from build123d import *

# Parameters (mm, degrees)
F0_R     = 6.5
F1_DEPTH = 50
F2_R     = 5.75
F3_DEPTH = 15
F4_R     = 4
F5_DEPTH = 4.5
F6_R     = 1


with BuildPart() as f1:
    # F0 (on Front) → F1 (new body)
    with BuildSketch(Plane.XZ):
        Circle(F0_R)
    extrude(amount=F1_DEPTH)

    # F2 (on face) → F3 (join)
    with BuildSketch(Plane.XZ.offset(50)):
        Circle(F2_R)
    extrude(amount=F3_DEPTH)

    # F4 (on face) → F5 (join)
    with BuildSketch(Plane.XZ.offset(65)):
        Circle(F4_R)
    extrude(amount=F5_DEPTH)

    # F6
    f6_edges = [f1.edges().sort_by_distance(p)[0] for p in [
        (-4, -69.5, 0),
        (-5.75, -65, 0),
        (-6.5, 0, 0),
    ]]
    fillet(f6_edges, radius=F6_R)


solid = f1.part
Input: part model. Units: mm. Frame: model coordinates. Give positions to 0.01 mm unless a question says otherwise; leave off trailing zeros. Loops run counter-clockwise (first coordinate to the right, second up) from the corner with the lowest first, then second, coordinate; pieces in that order, holes last. Notation, with made-up numbers: (42.5, -26.75) -> (89.5, -26.75) arc R20 ccw to (89.5, -12.75) -> close; hole circle Ø1 at (25, 27). An arc over 180 degrees is marked (long way). Answer as a JSON object with one key per item and string values. Group by question number.
Item 1: Line query: probe 1 along Y at (x, z) = (-4, 2.75); probe 2 along Z at (x, y) = (0, -63.5); probe 3 along Z at (x, y) = (-3.25, -62.5). Output: solid intervals per line, ascending.
Item 2: Pin query (flat end, axial travel): P1, Ø5, axis at y = -33, z = 3, coming from the +X side; P2, Ø6, axis at x = -1, z = -5, coming from the +Y side; P3, Ø1, axis at y = -20, z = -5, coming from the +X side; P4, Ø1, axis at x = 4.5, z = 4, coming from the -Y side. Return the tip coordinate at first contact, or that it passes through.
Item 3: Cut plane B-B, the plane y = -4. Return the cut outline in (x, z), and give its area (3 significant figures).
Item 4: Cut plane A-A, the plane x = 0. Return the cut outline in (y, z).
Item 5: Pull-direction query (Y, two-part tool) for faces 1 (the flat face through (0, 0, 0)), 2 (the cylindrical face through (-5.158, -25.157, -3.955)), 3 (the flat face through (0, -69.5, 0)); classes: released by +Y, released by -Y, zero draft, split by the parting line, or undercut.
Checks:
{
 "1": {"probe 1": "y = -64.99 to 0", "probe 2": "z = -5.75 to 5.75", "probe 3": "z = -4.74 to 4.74"},
 "2": {"P1": "stops at x = 6.48", "P2": "stops at y = 0", "P3": "stops at x = 4.69", "P4": "stops at y = -64.64"},
 "3": {"outline": "circle Ø13 at (0, 0)", "area": "133 mm²"},
 "4": {"outline": "(-69.5, -3) arc R1 ccw to (-68.5, -4) -> (-65, -4) -> (-65, -4.75) arc R1 ccw to (-64, -5.75) -> (-50, -5.75) -> (-50, -6.5) -> (-1, -6.5) arc R1 ccw to (0, -5.5) -> (0, 5.5) arc R1 ccw to (-1, 6.5) -> (-50, 6.5) -> (-50, 5.75) -> (-64, 5.75) arc R1 ccw to (-65, 4.75) -> (-65, 4) -> (-68.5, 4) arc R1 ccw to (-69.5, 3) -> close"},
 "5": {"face 1": "released by +Y", "face 2": "zero draft", "face 3": "released by -Y"}
}
